Model file for the job. Use its own axes, mm. Face numbers are marked on the shaded views. Coordinates: 2 decimals unless noted, no trailing zeros. Write each loop counter-clockwise with the first axis right and the second up, starting at its lowest first coordinate (ties: lowest second). Pieces come first, ordered by that corner, then holes.
Q1. Band-saw the part on A-A, the plane z = 16. Write the cut outline in (x, y), plus the area to 3 significant figures.
Q2. Band-saw the part on C-C, the plane y = -2.65. State how many separate pieces and enclosed holes the cut face has, plus the area to 3 significant figures.
Q3. Drill centre lines: probe 1 along X at (y, z) = (-2.8, -15); probe 2 along Z at (x, y) = (-84.5, -4.35) (3 decimals); probe 3 along Z at (x, y) = (-58, -2.1) (3 decimals). Where is each one in solid material? Low to high.
Q4. Pull direction Y, two halves, no side cores. Call the marked faces 1 and 2: released by +Y, released by -Y, zero draft, split by the parting line, or undercut.
Q5. Band-saw the part on B-B, the plane x = -31. Write the cut outline in (y, z) (3 decimals), plus the area to 3 significant figures.
Q6. Pin check, flat tips, straight feed: P1, Ø2.5, axis at x = 25, y = -3.5, coming from the -Z side; P2, Ø1.5, axis at y = -3, z = -32, coming from the +X side. Stop position of each tip, or through.
from build123d import *

# Parameters (mm, degrees)
F0_W     = 203.2
F0_H     = 69.85
F1_DEPTH = 5.207
F2_R     = 5.08
F3_W     = 5.207
F3_H     = 12.7
F3_W_2   = 12.7
F3_H_2   = 5.129387
F3_W_3   = 18.097754
F4_DEPTH = 5.208


with BuildPart() as f1:
    # F0 (on Front) → F1 (new body)
    with BuildSketch(Plane.XZ):
        Rectangle(F0_W, F0_H)
    extrude(amount=F1_DEPTH)

    # F2
    f2_edges = [f1.edges().sort_by_distance(p)[0] for p in [
        (-101.6, -2.6035, 34.925),
        (-101.6, -2.6035, -34.925),
        (101.6, -2.6035, -34.925),
        (101.6, -2.6035, 34.925),
    ]]
    fillet(f2_edges, radius=F2_R)

    # F3 (on face) → F4 (cut, through all)
    with BuildSketch(Plane.XZ.offset(5.207)):
        with Locations((-82.0166, 12.622387)):
            Rectangle(F3_W, F3_H)
        with Locations((-82.0166, -12.777613)):
            Rectangle(F3_W, F3_H)
        Polygon((-63.380809, -34.925), (-45.438314, -34.925), (-45.438314, -29.795613), (-63.39332, -29.795613), align=None)
        with Locations((-26.388314, -32.360307)):
            Rectangle(F3_W_2, F3_H_2)
        with Locations((-0.988314, -32.360307)):
            Rectangle(F3_W_2, F3_H_2)
        with Locations((24.411686, -32.360307)):
            Rectangle(F3_W_2, F3_H_2)
        with Locations((52.510563, -32.360307)):
            Rectangle(F3_W_3, F3_H_2)
        with Locations((82.0166, -12.777613)):
            Rectangle(F3_W, F3_H)
        with Locations((82.0166, 12.622387)):
            Rectangle(F3_W, F3_H)
    extrude(amount=-F4_DEPTH, mode=Mode.SUBTRACT)


solid = f1.part
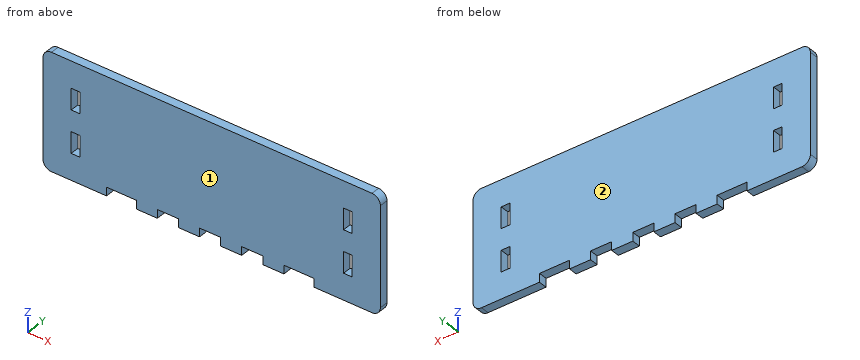
Answer sheet:
1. outline: (-101.6, -5.21) - (-84.62, -5.21) - (-84.62, 0) - (-101.6, 0) - close; (-79.41, -5.21) - (79.41, -5.21) - (79.41, 0) - (-79.41, 0) - close; (84.62, -5.21) - (101.6, -5.21) - (101.6, 0) - (84.62, 0) - close
1. area: 1,000 mm2
2. separate pieces: 1
2. enclosed holes: 4
2. area: 13,500 mm2
3. probe 1: x = -101.6 to -84.62, -79.41 to 79.41, 84.62 to 101.6
3. probe 2: z = -34.925 to -19.128, -6.428 to 6.272, 18.972 to 34.925
3. probe 3: z = -29.796 to 34.925
4. face 1: released by -Y
4. face 2: released by +Y
5. outline: (-5.207, -29.796) - (0, -29.796) - (0, 34.925) - (-5.207, 34.925) - close
5. area: 337 mm2
6. P1: stops at z = -29.8
6. P2: stops at x = 101.4
